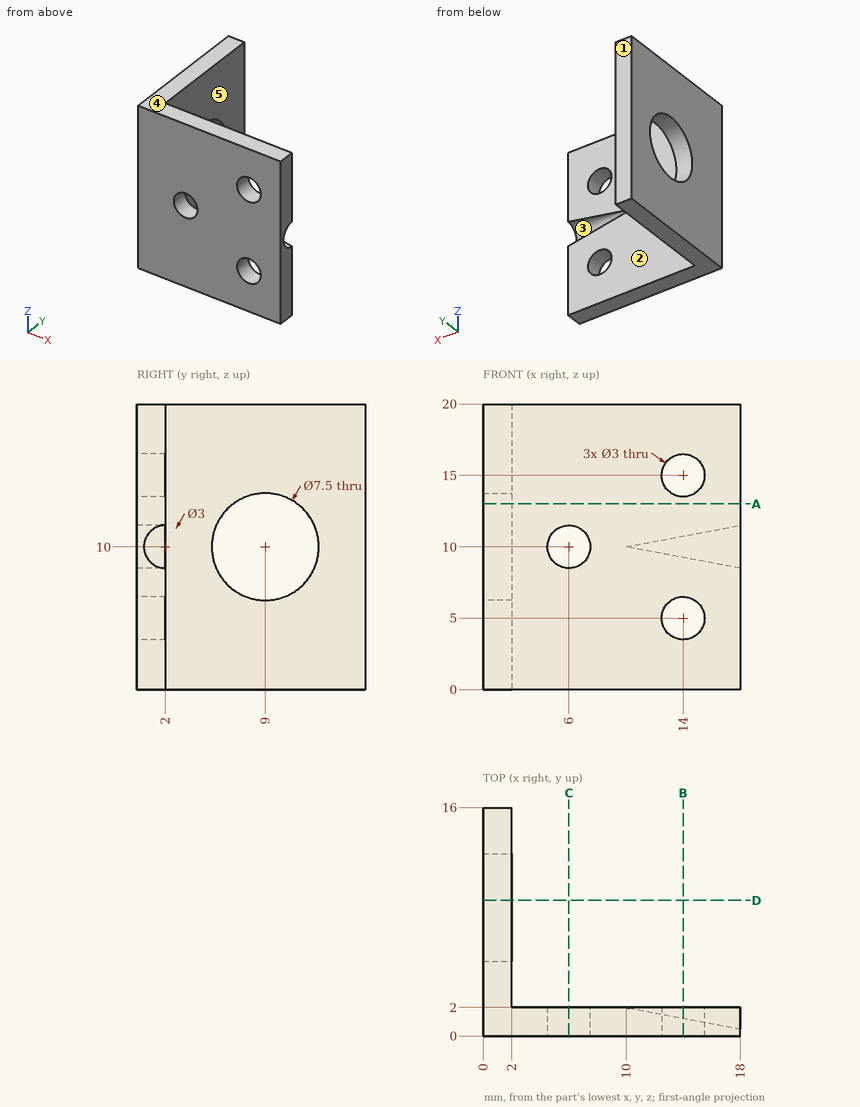
Verification items for this drawing (mm, ordinates from the low corner). A direction names the side the tool comes from. Give positions to 0.01 mm unless a question says otherwise; leave off trailing zeros. Loops run counter-clockwise (first coordinate to the right, second up) from the corner with the lowest first, then second, coordinate; pieces in that order, holes last. Notation, with made-up numbers: (64, 64) - (105, 64) arc R20 ccw to (105, 70) - close; hole circle Ø7 at (15.5, 66.5). An arc over 180 degrees is marked (long way). Write item = value, one per line. Start each with the question number.
Q1. Mould release check, pull along Z, two halves, no side actions. Record for the marked faces 3, 4 and 5: released by +Z, released by -Z, zero draft, split by the parting line, or undercut.
Q2. Depth check by flat-ended pin: P1, Ø5, axis at y = 12.5, z = 17.5, coming from the +X side; P2, Ø4, axis at x = 12, z = 9, coming from the +Y side. Enter the tip coordinate at first touch or a pass-through.
Q3. Cross-section at D-D, the plane y = 9.5. Enter the section's corners in (x, z), and give its area (3 significant figures).
Q4. Cross-section at A-A, the plane z = 13. Enter the section's corners in (x, y), and give its area (3 significant figures).
Q5. Thickness scan on line 1 (X direction, y = 0.5, z = 5); line 2 (Y direction, x = 0.6, z = 10); line 3 (Z direction, x = 14, y = 0.95). Record the ranges inside material, lowest first.
Q6. Cross-section at B-B, the plane x = 14. Enter the section's corners in (y, z), and give its area (3 significant figures).
Q7. Tool access check on the marked faces 1 and 2. Record the directions out of +Z, -Z, +X, -X, +Y, -Y that give a thin tool (end or side, any length) a straight path to the whole face; none if there is none.
Q8. Cross-section at C-C, the plane x = 6. Enter the section's corners in (y, z), and give its area (3 significant figures).
Answer key:
q1.face_3 = undercut
q1.face_4 = released by +Z
q1.face_5 = zero draft
q2.P1 = 2
q2.P2 = 2
q3.outline = (0, 0) - (2, 0) - (2, 6.28) - (0, 6.28) - close; (0, 13.72) - (2, 13.72) - (2, 20) - (0, 20) - close
q3.area = 25.1 mm^2
q4.outline = (0, 0) - (18, 0) - (18, 2) - (2, 2) - (2, 6.75) - (0, 6.75) - close; (0, 11.25) - (2, 11.25) - (2, 16) - (0, 16) - close
q4.area = 55.0 mm^2
q5.line_1 = 0 to 12.5, 15.5 to 18
q5.line_2 = 0 to 5.25, 12.75 to 16
q5.line_3 = 0 to 3.5, 6.5 to 13.5, 16.5 to 20
q6.outline = (0, 0) - (2, 0) - (2, 3.5) - (0, 3.5) - close; (0, 6.5) - (2, 6.5) - (2, 9.25) arc R0.75 cw to (2, 10.75) - (2, 13.5) - (0, 13.5) - close; (0, 16.5) - (2, 16.5) - (2, 20) - (0, 20) - close
q6.area = 27.1 mm^2
q7.face_1 = +Z, -Z, +X, -X, +Y
q7.face_2 = +Z, -Z, +X, +Y
q8.outline = (0, 0) - (2, 0) - (2, 8.5) - (0, 8.5) - close; (0, 11.5) - (2, 11.5) - (2, 20) - (0, 20) - close
q8.area = 34.0 mm^2
